```python
from build123d import *

# Parameters (mm, degrees)
SKETCH1_R           = 45
SKETCH1_R_2         = 2.75
SKETCH1_R_3         = 1.25
BOSS_EXTRUDE1_DEPTH = 12.7
SKETCH2_R           = 17.75
CUT_EXTRUDE1_DEPTH  = 6.35
SKETCH3_R           = 6
CUT_EXTRUDE2_DEPTH  = 64.95562915
SKETCH4_R           = 28.5
CUT_EXTRUDE3_DEPTH  = 6.35
SKETCH6_R           = 4.25
CUT_EXTRUDE4_DEPTH  = 6.35


with BuildPart() as part:
    # Sketch1 → Boss-Extrude1 (new body)
    with BuildSketch(Plane(origin=(0, 0, 0), x_dir=(1, 0, 0), z_dir=(0, 1, 0))):
        with Locations(Location((0, 0, 0), (0, 0, 270))):
            Circle(SKETCH1_R)
        with Locations(Location((0, 32.5, 0), (0, 0, 270))):
            Circle(SKETCH1_R_2, mode=Mode.SUBTRACT)
        with Locations(Location((28.145825623, -16.25, 0), (0, 0, 270))):
            Circle(SKETCH1_R_2, mode=Mode.SUBTRACT)
        with Locations(Location((-28.145825623, -16.25, 0), (0, 0, 270))):
            Circle(SKETCH1_R_2, mode=Mode.SUBTRACT)
        with Locations(Location((-36.435998127, -7.744710483, 0), (0, 0, 270))):
            Circle(SKETCH1_R_3, mode=Mode.SUBTRACT)
        with Locations(Location((-34.029568297, 15.150939955, 0), (0, 0, 270))):
            Circle(SKETCH1_R_3, mode=Mode.SUBTRACT)
        with Locations(Location((-18.625, 32.259446291, 0), (0, 0, 270))):
            Circle(SKETCH1_R_3, mode=Mode.SUBTRACT)
        with Locations(Location((3.893685257, 37.045940602, 0), (0, 0, 270))):
            Circle(SKETCH1_R_3, mode=Mode.SUBTRACT)
        with Locations(Location((24.925115087, 27.682144749, 0), (0, 0, 270))):
            Circle(SKETCH1_R_3, mode=Mode.SUBTRACT)
        with Locations(Location((36.435998127, 7.744710483, 0), (0, 0, 270))):
            Circle(SKETCH1_R_3, mode=Mode.SUBTRACT)
        with Locations(Location((34.029568297, -15.150939955, 0), (0, 0, 270))):
            Circle(SKETCH1_R_3, mode=Mode.SUBTRACT)
        with Locations(Location((18.625, -32.259446291, 0), (0, 0, 270))):
            Circle(SKETCH1_R_3, mode=Mode.SUBTRACT)
        with Locations(Location((-3.893685257, -37.045940602, 0), (0, 0, 270))):
            Circle(SKETCH1_R_3, mode=Mode.SUBTRACT)
        with Locations(Location((-24.925115087, -27.682144749, 0), (0, 0, 270))):
            Circle(SKETCH1_R_3, mode=Mode.SUBTRACT)
    extrude(amount=BOSS_EXTRUDE1_DEPTH)

    # Sketch2 → Cut-Extrude1 (cut)
    with BuildSketch(Plane(origin=(0, 12.7, 0), x_dir=(1, 0, 0), z_dir=(0, 1, 0))):
        with Locations(Location((0, 0, 0), (0, 0, 270))):
            Circle(SKETCH2_R)
    extrude(amount=-CUT_EXTRUDE1_DEPTH, mode=Mode.SUBTRACT)

    # Sketch3 → Cut-Extrude2 (cut, through all)
    with BuildSketch(Plane(origin=(0, 6.35, 0), x_dir=(1, 0, 0), z_dir=(0, 1, 0))):
        with Locations(Location((0, 0, 0), (0, 0, 270))):
            Circle(SKETCH3_R)
    extrude(amount=-CUT_EXTRUDE2_DEPTH, mode=Mode.SUBTRACT)

    # Sketch4 → Cut-Extrude3 (cut)
    with BuildSketch(Plane.XZ):
        with Locations(Location((0, 0, 0), (0, 0, 270))):
            Circle(SKETCH4_R)
    extrude(amount=-CUT_EXTRUDE3_DEPTH, mode=Mode.SUBTRACT)

    # Sketch6 → Cut-Extrude4 (cut)
    with BuildSketch(Plane.XZ):
        with Locations((28.145825623, 16.25)):
            Circle(SKETCH6_R)
        with Locations((0, -32.5)):
            Circle(SKETCH6_R)
        with Locations((-28.145825623, 16.25)):
            Circle(SKETCH6_R)
    extrude(amount=-CUT_EXTRUDE4_DEPTH, mode=Mode.SUBTRACT)


solid = part.part
```
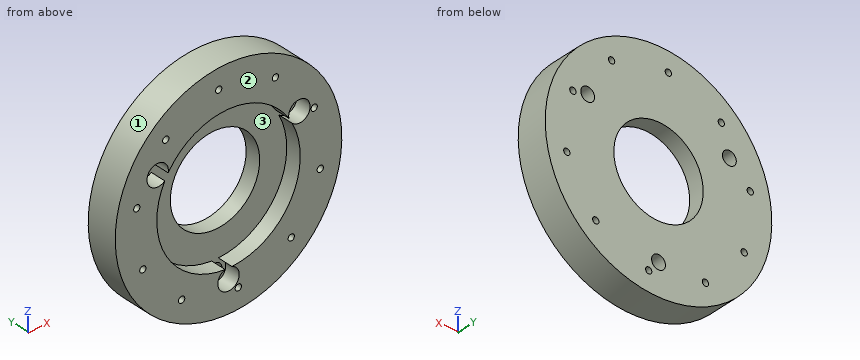
Geometry: final body of the model. Coordinates: model frame, mm. Face numbers are marked on the shaded views. Give positions to 0.01 mm unless a question says otherwise; leave off trailing zeros. Write each loop counter-clockwise with the first axis right and the second up, starting at its lowest first coordinate (ties: lowest second). Pieces come first, ordered by that corner, then holes.
1. Section query C-C, the plane y = 9.75. Count the separate pieces of the cut face and the enclosed holes in it, then the cut area to 3 significant figures.
2. Pin query (flat end, axial travel): P1, Ø6, axis at x = -34, y = 10.5, coming from the -Z side; P2, Ø2, axis at x = -36.44, z = 7.74, coming from the +Y side; P3, Ø7, axis at x = -28.15, z = 16.25, coming from the -Y side; P4, Ø4, axis at y = 9.5, z = -36, coming from the +X side. Return the tip coordinate at first contact, or that it passes through.
3. Section query B-B, the plane z = 0. Return loops of the section in (x, y), then the cut area to 3 significant figures.
4. Section query D-D, the plane x = -15.5. Return loops of the section in (y, z).
5. Line query: probe 1 along Z at (x, y) = (3, 10.25); probe 2 along Z at (x, y) = (15.5, 2.75); probe 3 along Z at (x, y) = (15.5, 12). Output: solid intervals per line, ascending.
6. Section query A-A, the plane x = 0. Return loops of the section in (y, z), then the cut area to 3 significant figures.
7. Draft query along Z for the marked faces 1, 2 and 3. Return one class per face: released by +Z, released by -Z, zero draft, split by the parting line, or undercut.
Computed:
1. separate pieces: 1
1. enclosed holes: 14
1. area: 5,250 mm2
2. P1: stops at z = -32.62
2. P2: passes through
2. P3: stops at y = 6.35
2. P4: stops at x = 29.48
3. outline: (-45, 0) - (-28.5, 0) - (-28.5, 6.35) - (-17.75, 6.35) - (-17.75, 12.7) - (-45, 12.7) - close; (17.75, 6.35) - (28.5, 6.35) - (28.5, 0) - (45, 0) - (45, 12.7) - (17.75, 12.7) - close
3. area: 556 mm2
4. outline: (0, -42.25) - (12.7, -42.25) - (12.7, -8.65) - (6.35, -8.65) - (6.35, -23.92) - (0, -23.92) - close; (0, 23.92) - (6.35, 23.92) - (6.35, 8.65) - (12.7, 8.65) - (12.7, 42.25) - (0, 42.25) - close
5. probe 1: z = -44.9 to -37.92, -36.17 to -17.49, 17.49 to 44.9
5. probe 2: z = -42.25 to -23.92, 23.92 to 42.25
5. probe 3: z = -42.25 to -8.65, 8.65 to 42.25
6. outline: (0, -45) - (12.7, -45) - (12.7, -35.25) - (6.35, -35.25) - (6.35, -36.75) - (0, -36.75) - close; (0, 28.5) - (6.35, 28.5) - (6.35, 17.75) - (12.7, 17.75) - (12.7, 45) - (0, 45) - close; (6.35, -29.75) - (12.7, -29.75) - (12.7, -17.75) - (6.35, -17.75) - close
6. area: 468 mm2
7. face 1: split by the parting line
7. face 2: zero draft
7. face 3: undercut
